The listing builds one solid part. Answer for the finished solid, in the listing's coordinates (mm). A direction names the side the tool comes from. Coordinates: 2 decimals unless noted, no trailing zeros. Order: outer loops, then holes, each group sorted by start corner. A loop starts at its lowest first (then second) coordinate and runs counter-clockwise, first axis right, second up.
Autodesk Inventor part; units mm, degrees
ref_plane "YZ Plane" through (0, 0, 0) normal (1, 0, 0) x (0, 1, 0)
ref_plane "XZ Plane" through (0, 0, 0) normal (0, 1, 0) x (-1, 0, 0)
ref_plane "XY Plane" through (0, 0, 0) normal (0, 0, 1) x (1, 0, 0)
sketch "草圖2" plane through (0, 0, 0) normal (0, 0, 1) x (1, 0, 0)
  circle A0 centre (0, 0) radius 177.5
  dimension "d8" = 355
extrude "擠出2" add sketch "草圖2" against normal blind 10
sketch "草圖1" plane through (0, 0, 0) normal (0, 0, 1) x (1, 0, 0)
  circle A0 centre (150, 0) radius 9
  circle A1 centre (144.8889, 38.8229) radius 9
  circle A2 centre (129.9038, 75) radius 9
  circle A3 centre (106.066, 106.066) radius 9
  circle A4 centre (75, 129.9038) radius 9
  circle A5 centre (38.8229, 144.8889) radius 9
  circle A6 centre (0, 150) radius 9
  circle A7 centre (-38.8229, 144.8889) radius 9
  circle A8 centre (-75, 129.9038) radius 9
  circle A9 centre (-106.066, 106.066) radius 9
  circle A10 centre (-129.9038, 75) radius 9
  circle A11 centre (-144.8889, 38.8229) radius 9
  circle A12 centre (-150, 0) radius 9
  circle A13 centre (-144.8889, -38.8229) radius 9
  circle A14 centre (-129.9038, -75) radius 9
  circle A15 centre (-106.066, -106.066) radius 9
  circle A16 centre (-75, -129.9038) radius 9
  circle A17 centre (-38.8229, -144.8889) radius 9
  circle A18 centre (0, -150) radius 9
  circle A19 centre (38.8229, -144.8889) radius 9
  circle A20 centre (75, -129.9038) radius 9
  circle A21 centre (106.066, -106.066) radius 9
  circle A22 centre (129.9038, -75) radius 9
  circle A23 centre (144.8889, -38.8229) radius 9
  point P0 (0, 0)
  dimension "d0" = 150
  dimension "d1" = 18
  dimension "d4" = 360
extrude "擠出3" cut sketch "草圖1" against normal blind 5
sketch "草圖3" plane through (0, 0, 0) normal (0, 0, 1) x (1, 0, 0)
  circle A0 centre (0, 0) radius 75
  dimension "d13" = 150
extrude "擠出4" cut sketch "草圖3" against normal blind 10
properties part number "pindisk"
(1) For faces 1 (the face through (75, -130, -5)), 2 (the face through (-9.764, 74.362, -4.93)), determine the directions among +Z, -Z, +X, -X, +Y, -Y from which every point of the face is accessible in a straight line to the end or side of a thin tool.
(2) Find section C-C (z = -1.75). Give the number of separate pieces and of enclosed holes in the cut face, and give its area (3 significant figures).
(3) Consider line 1 (Y direction, x = 38, z = -2.25); line 2 (Y direction, x = 150, z = -2.2); line 3 (X direction, y = -37, z = -2.25). Determine where each line is inside the solid, lowest interval first.
(4) Find section D-D (x = 129.5). Write down the section's boundary in (y, z).
(5) Each of these flat-tipped pins is pushed along its axis until it touches: pin 1 Ø3 at (y, z) = (7, -5.5) entering from +X; pin 2 Ø14.5 at (x, y) = (152.5, 3) entering from +Z; pin 3 Ø5.5 at (x, y) = (-149.5, -0.5) entering from +Z; pin 4 Ø3 at (y, z) = (-28, -4) entering from +X. Where does it stop, or does it pass through?
(6) Find section B-B (x = -52.5). Write down the section's boundary in (y, z).
(7) The mould has two halves that part along X. Classify faces 3 (the face through (-101.91, -114.05, -2.46)), 4 (the face through (-130, 75, -5)): released by +X, released by -X, zero draft, split by the parting line, or undercut.
(8) Find section A-A (y = 4.5). Write down the section's boundary in (x, z).
Findings below:
1. face 1: +Z
1. face 2: +Z, -Z
2. separate pieces: 1
2. enclosed holes: 25
2. area: 75,200 mm2
3. line 1: y = -173.38 to -153.85, -135.93 to -64.66, 64.66 to 135.93, 153.85 to 173.38
3. line 2: y = -94.9 to -46.23, -31.42 to -9, 9 to 31.42, 46.23 to 94.9
3. line 3: x = -173.6 to -153.7, -136.08 to -65.24, 65.24 to 136.08, 153.7 to 173.6
4. outline: (-121.39, -10) - (121.39, -10) - (121.39, 0) - (83.99, 0) - (83.99, -5) - (66.01, -5) - (66.01, 0) - (-66.01, 0) - (-66.01, -5) - (-83.99, -5) - (-83.99, 0) - (-121.39, 0) - close
5. pin 1: stops at x = 177.41
5. pin 2: stops at z = 0
5. pin 3: stops at z = -5
5. pin 4: stops at x = 175.51
6. outline: (-169.56, -10) - (-53.56, -10) - (-53.56, 0) - (-169.56, 0) - close; (53.56, -10) - (169.56, -10) - (169.56, 0) - (53.56, 0) - close
7. face 3: undercut
7. face 4: undercut
8. outline: (-177.44, -10) - (-74.86, -10) - (-74.86, 0) - (-142.21, 0) - (-142.21, -5) - (-157.79, -5) - (-157.79, 0) - (-177.44, 0) - close; (74.86, -10) - (177.44, -10) - (177.44, 0) - (157.79, 0) - (157.79, -5) - (142.21, -5) - (142.21, 0) - (74.86, 0) - close
